Autodesk Fusion 360 part; units mm, degrees
sketch "Szkic1" plane through (0, 0, 0) normal (1, 0, 0) x (0, 1, 0)
  line L0 (8, 25) -> (12, 25)
  line L1 (20, 17) -> (20, -5)
  line L2 (12, -13) -> (8, -13)
  line L3 (0, -5) -> (0, 17)
  arc A0 (8, 25) -> (0, 17) centre (8, 17) ccw
  arc A1 (20, 17) -> (12, 25) centre (12, 17) ccw
  arc A2 (12, -13) -> (20, -5) centre (12, -5) ccw
  arc A3 (0, -5) -> (8, -13) centre (8, -5) ccw
  point P0 (0, 25)
  point P1 (20, 25)
  point P2 (20, -13)
  dimension "d1" = 20
  dimension "d2" = 38
  dimension "d3" = 8
  dimension "d4" = 8
extrude "Wyciągnięcie proste1" add sketch "Szkic1" along normal blind 132
Build history of the part. All positions in model axes, mm. Give positions to 0.01 mm unless a question says otherwise; leave off trailing zeros. Order: outer loops, then holes, each group sorted by start corner. A loop starts at its lowest first (then second) coordinate and runs counter-clockwise, first axis right, second up. Notation, with made-up numbers: M 87,30 L 132,30 A21 ccw 132,40 Z; hole C 4.5,45.25 d4. An arc over 180 degrees is marked long. Write item = value, one per line. Start each with the question number.
(1) Probe L1, parallel to Z at x = 29.5, y = 5.5; L2, parallel to Y at x = 122, z = -7; L3, parallel to Y at x = 103.5, z = -6. List the from-to ranges inside material, lowest first. Write a range as [from, to].
(2) Slice it at A-A on x = 67.5. Write the cut outline in (y, z).
(3) Pin check, flat tips, straight feed: pin 1 Ø5 at (y, z) = (11.5, 2.5) entering from -X; pin 2 Ø2 at (x, y) = (77.5, 6.5) entering from -Z; pin 3 Ø6 at (x, y) = (71, 16) entering from +Z. Stop position of each tip, or through.
(4) Slice it at B-B on y = 1.5. Write the cut outline in (x, z).
(5) Slice it at C-C on z = -8.5. Write the cut outline in (x, y).
Responses:
q1.L1 = [-12.6, 24.6]
q1.L2 = [0.25, 19.75]
q1.L3 = [0.06, 19.94]
q2.outline = M 0,-5 A8 ccw 8,-13 L 12,-13 A8 ccw 20,-5 L 20,17 A8 ccw 12,25 L 8,25 A8 ccw 0,17 Z
q3.pin_1 = 0
q3.pin_2 = -12.98
q3.pin_3 = 24.94
q4.outline = M 0,-9.66 L 132,-9.66 L 132,21.66 L 0,21.66 Z
q5.outline = M 0,0.81 L 132,0.81 L 132,19.19 L 0,19.19 Z
